Autodesk Inventor part; units mm, degrees
ref_plane "YZ Plane" through (0, 0, 0) normal (1, 0, 0) x (0, 1, 0)
ref_plane "XZ Plane" through (0, 0, 0) normal (0, 1, 0) x (-1, 0, 0)
ref_plane "XY Plane" through (0, 0, 0) normal (0, 0, 1) x (1, 0, 0)
sketch "Szkic1" plane through (0, 0, 0) normal (0, 0, 1) x (1, 0, 0)
  line L0 (-30, -35) -> (30, -35)
  line L1 (30, -35) -> (30, 35)
  line L2 (30, 35) -> (-30, 35)
  line L3 (-30, 35) -> (-30, -35)
  line L4 (-30, -35) -> (30, 35) construction
  line L5 (30, -35) -> (-30, 35) construction
  point P0 (0, 0)
  dimension "d0" = 60
  dimension "d1" = 70
extrude "Wyciągnięcie proste1" add sketch "Szkic1" along normal blind 8
sketch "Szkic2" plane through (0, 0, 0) normal (0, 0, -1) x (-1, 0, 0)
  line L0 (30, -35) -> (-30, -35)
  line L1 (30, 35) -> (30, -35)
  line L2 (-30, 35) -> (30, 35)
  line L3 (-30, -35) -> (-30, 35)
  line L4 (23.57, 5) -> (23.57, 28.57)
  line L5 (23.57, 28.57) -> (-23.57, 28.57)
  line L6 (-23.57, 28.57) -> (-23.57, -18.57)
  line L7 (-23.57, -18.57) -> (23.57, -18.57)
  line L8 (23.57, -18.57) -> (23.57, 5)
  circle A0 centre (23.57, 28.57) radius 2.5
  circle A1 centre (-23.57, 28.57) radius 2.5
  circle A2 centre (-23.57, -18.57) radius 2.5
  circle A3 centre (23.57, -18.57) radius 2.5
  line L9 (0, 0) -> (0, 5)
  dimension "d6" = 47.14
  dimension "d7" = 47.14
  dimension "d8" = 47.14
  dimension "d9" = 5
  dimension "d10" = 5
  dimension "d11" = 5
  dimension "d12" = 5
  dimension "d15" = 5
extrude "Wyciągnięcie proste3" cut sketch "Szkic2" against normal up to next contours A0 L5 L4 | L4 L5 A0 | A3 L7 L8 | L8 L7 A3 | A1 L6 L5 | L5 L6 A1 | A2 L6 L7 | L7 L6 A2
sketch "Szkic4" plane through (0, 0, 8) normal (0, 0, 1) x (1, 0, 0)
  line L0 (-30, -35) -> (30, -35)
  line L1 (30, -35) -> (30, -43)
  line L2 (30, -43) -> (-30, -43)
  line L3 (-30, -43) -> (-30, -35)
  point P0 (0, 0)
  dimension "d18" = 8
extrude "Wyciągnięcie proste4" add sketch "Szkic4" against normal blind 43.4
sketch "Szkic5" plane through (0, 0, 8) normal (0, 0, 1) x (1, 0, 0)
  circle A0 centre (-23.57, -18.57) radius 2.5
  circle A1 centre (23.57, 28.57) radius 2.5
  circle A2 centre (-23.57, 28.57) radius 2.5
  circle A3 centre (23.57, -18.57) radius 2.5
  line L0 (30, 35) -> (30, -43)
  line L1 (30, 35) -> (-30, 35)
  line L2 (-30, 35) -> (-30, -43)
  line L3 (30, -43) -> (-30, -43)
  line L4 (23.57, -18.57) -> (-23.57, 28.57)
  line L5 (-23.57, -18.57) -> (23.57, 28.57)
  circle A4 centre (0, 5) radius 15
  point P0 (0, 0)
  dimension "d21" = 30
extrude "Wyciągnięcie proste5" cut sketch "Szkic5" against normal up to next contours A4 L4 L5 | L5 L4 A4 | L5 A4 L4 | L4 A4 L5
thread "Gwint1"
thread "Gwint2"
thread "Gwint3"
thread "Gwint4"
sketch "Szkic10" plane through (0, 0, 0) normal (0, 0, -1) x (-1, 0, 0)
  circle A0 centre (0, 5) radius 15
  circle A1 centre (0, 5) radius 19.5
  point P0 (0, 0)
  dimension "d59" = 39
extrude "Wyciągnięcie proste10" cut sketch "Szkic10" against normal blind 2
sketch "Szkic12" plane through (0, 0, -35.4) normal (0, 0, -1) x (-1, 0, 0)
  line L0 (30, -35) -> (-30, -35)
  line L1 (-30, -35) -> (-30, -43)
  line L2 (-30, -43) -> (30, -43)
  line L3 (30, -43) -> (30, -35)
  point P0 (0, 0)
extrude "Wyciągnięcie proste12" cut sketch "Szkic12" against normal blind 20
sketch "Szkic13" plane through (-30, -43, 8) normal (0, -1, 0) x (1, 0, 0)
  line L0 (0, -23.4) -> (60, -23.4)
  line L1 (0, 0) -> (0, -23.4)
  line L2 (60, 0) -> (60, -23.4)
  line L3 (60, -23.4) -> (60, -15.4)
  line L4 (60, -8) -> (60, -23.4)
  line L5 (60, -15.4) -> (0, -15.4)
  point P0 (30, -8)
  dimension "d66" = 8
extrude "Wyciągnięcie proste13" add sketch "Szkic13" along normal blind 60
sketch "Szkic16" plane through (-30, -43, -7.4) normal (0, 0, 1) x (1, 0, 0)
  line L0 (60, -60) -> (0, -60)
  line L1 (60, 0) -> (60, -60)
  line L2 (0, 0) -> (60, 0)
  line L3 (0, 0) -> (0, -60)
  circle A0 centre (30, -20) radius 6.5
  line L4 (30, -20) -> (35, -20)
  line L5 (30, -20) -> (25, -20)
  arc A1 (35, -30) -> (35, -10) centre (35, -20) ccw
  arc A2 (25, -10) -> (25, -30) centre (25, -20) ccw
  line L6 (25, -10) -> (35, -10)
  line L7 (35, -30) -> (25, -30)
  point P0 (30, 43)
  dimension "d87" = 5
  dimension "d88" = 5
  dimension "d89" = 10
extrude "Wyciągnięcie proste15" cut sketch "Szkic16" against normal up to next contours A0 | L7 A2 L6 A1
sketch "Szkic17" plane through (-30, -43, -7.4) normal (0, 0, 1) x (1, 0, 0)
  line L0 (25, -10) -> (35, -10)
  arc A0 (35, -30) -> (35, -10) centre (35, -20) ccw
  line L1 (35, -30) -> (25, -30)
  arc A1 (25, -10) -> (25, -30) centre (25, -20) ccw
  line L2 (0, 0) -> (60, 0)
  line L3 (0, 0) -> (0, -60)
  line L4 (60, -60) -> (0, -60)
  line L5 (60, 0) -> (60, -60)
  line L6 (60, 0) -> (60, -5)
  line L7 (60, 8) -> (60, -60)
  line L8 (30, -30) -> (30, -35)
  line L9 (60, -5) -> (57.5, -5)
  arc A2 (55, -7.5) -> (55, -2.5) centre (55, -5) ccw
  arc A3 (45, -2.5) -> (45, -7.5) centre (45, -5) ccw
  line L10 (55, -7.5) -> (45, -7.5)
  line L11 (60, -5) -> (57.5, -5)
  line L12 (55, -2.5) -> (45, -2.5)
  line L13 (60, -35) -> (57.5, -35)
  arc A4 (55, -37.5) -> (55, -32.5) centre (55, -35) ccw
  arc A5 (45, -32.5) -> (45, -37.5) centre (45, -35) ccw
  line L14 (55, -37.5) -> (45, -37.5)
  line L15 (55, -32.5) -> (45, -32.5)
  line L16 (30, -35) -> (42.5, -35)
  line L17 (57.5, -35) -> (60, -35)
  line L18 (0, -5) -> (2.5, -5)
  line L19 (0, -35) -> (2.5, -35)
  arc A6 (15, -7.5) -> (15, -2.5) centre (15, -5) ccw
  line L20 (15, -7.5) -> (5, -7.5)
  line L21 (15, -2.5) -> (5, -2.5)
  arc A7 (5, -2.5) -> (5, -7.5) centre (5, -5) ccw
  arc A8 (15, -37.5) -> (15, -32.5) centre (15, -35) ccw
  line L22 (15, -37.5) -> (5, -37.5)
  line L23 (15, -32.5) -> (5, -32.5)
  arc A9 (5, -32.5) -> (5, -37.5) centre (5, -35) ccw
  line L24 (42.5, -5) -> (17.5, -5)
  line L25 (2.5, -5) -> (0, -5)
  line L26 (30, -35) -> (17.5, -35)
  line L27 (2.5, -35) -> (0, -35)
  point P0 (30, 43)
  dimension "d92" = 5
  dimension "d93" = 5
  dimension "d98" = 2.5
  dimension "d99" = 2.5
  dimension "d100" = 2.5
  dimension "d101" = 2.5
extrude "Wyciągnięcie proste16" cut sketch "Szkic17" against normal up to next contours A5 L15 A4 L14 | A8 L22 A9 L23 | A2 L10 A3 L12 | A7 L21 A6 L20
sketch "Szkic18" plane through (-30, -43, -7.4) normal (0, 0, 1) x (1, 0, 0)
  line L0 (55, -5) -> (50, -5)
  line L1 (55, -35) -> (50, -35)
  line L2 (5, -5) -> (10, -5)
  line L3 (5, -35) -> (10, -35)
  circle A0 centre (10, -5) radius 2
  circle A1 centre (10, -35) radius 2
  circle A2 centre (50, -35) radius 2
  circle A3 centre (50, -5) radius 2
  line L4 (45, -2.5) -> (55, -2.5)
  arc A4 (55, -7.5) -> (55, -2.5) centre (55, -5) ccw
  line L5 (55, -7.5) -> (45, -7.5)
  arc A5 (45, -2.5) -> (45, -7.5) centre (45, -5) ccw
  line L6 (15, -37.5) -> (5, -37.5)
  arc A6 (5, -32.5) -> (5, -37.5) centre (5, -35) ccw
  line L7 (5, -32.5) -> (15, -32.5)
  arc A7 (15, -37.5) -> (15, -32.5) centre (15, -35) ccw
  line L8 (5, -2.5) -> (15, -2.5)
  arc A8 (15, -7.5) -> (15, -2.5) centre (15, -5) ccw
  line L9 (15, -7.5) -> (5, -7.5)
  arc A9 (5, -2.5) -> (5, -7.5) centre (5, -5) ccw
  line L10 (55, -37.5) -> (45, -37.5)
  arc A10 (45, -32.5) -> (45, -37.5) centre (45, -35) ccw
  line L11 (45, -32.5) -> (55, -32.5)
  arc A11 (55, -37.5) -> (55, -32.5) centre (55, -35) ccw
  line L12 (25, -10) -> (35, -10)
  arc A12 (35, -30) -> (35, -10) centre (35, -20) ccw
  line L13 (35, -30) -> (25, -30)
  arc A13 (25, -10) -> (25, -30) centre (25, -20) ccw
  line L14 (0, 0) -> (60, 0)
  line L15 (0, 0) -> (0, -60)
  line L16 (60, -60) -> (0, -60)
  line L17 (60, 0) -> (60, -60)
  line L18 (55, -5) -> (60, -5)
  line L19 (55, -35) -> (60, -35)
  line L20 (5, -5) -> (0, -5)
  line L21 (5, -35) -> (0, -35)
  point P0 (30, 43)
  dimension "d104" = 5
  dimension "d105" = 5
  dimension "d106" = 5
  dimension "d107" = 5
  dimension "d108" = 4
  dimension "d109" = 4
  dimension "d110" = 4
  dimension "d111" = 4
sketch "Szkic19" plane through (-30, -43, -7.4) normal (0, 0, 1) x (1, 0, 0)
  line L0 (45, -2.5) -> (55, -2.5)
  arc A0 (55, -7.5) -> (55, -2.5) centre (55, -5) ccw
  line L1 (55, -7.5) -> (45, -7.5)
  arc A1 (45, -2.5) -> (45, -7.5) centre (45, -5) ccw
  line L2 (15, -37.5) -> (5, -37.5)
  arc A2 (5, -32.5) -> (5, -37.5) centre (5, -35) ccw
  line L3 (5, -32.5) -> (15, -32.5)
  arc A3 (15, -37.5) -> (15, -32.5) centre (15, -35) ccw
  line L4 (5, -2.5) -> (15, -2.5)
  arc A4 (15, -7.5) -> (15, -2.5) centre (15, -5) ccw
  line L5 (15, -7.5) -> (5, -7.5)
  arc A5 (5, -2.5) -> (5, -7.5) centre (5, -5) ccw
  line L6 (55, -37.5) -> (45, -37.5)
  arc A6 (45, -32.5) -> (45, -37.5) centre (45, -35) ccw
  line L7 (45, -32.5) -> (55, -32.5)
  arc A7 (55, -37.5) -> (55, -32.5) centre (55, -35) ccw
  line L8 (25, -10) -> (35, -10)
  arc A8 (35, -30) -> (35, -10) centre (35, -20) ccw
  line L9 (35, -30) -> (25, -30)
  arc A9 (25, -10) -> (25, -30) centre (25, -20) ccw
  line L10 (0, 0) -> (60, 0)
  line L11 (60, -60) -> (0, -60)
  line L12 (60, 0) -> (60, -60)
  line L13 (60, 0) -> (60, -60)
  line L14 (60, -60) -> (0, -60)
  line L15 (0, 0) -> (60, 0)
  circle A10 centre (29.9999, -20) radius 6.5
  circle A11 centre (-10.0001, -20) radius 6.5
  line L16 (-10.0001, -20) -> (-5.0001, -20)
  arc A12 (0, -28.6602) -> (0, -11.3398) centre (-5.0001, -20) ccw
  line L17 (0, 0) -> (0, -2.5)
  line L18 (0, -37.5) -> (0, -60)
  line L19 (0, -11.3398) -> (0, -2.5)
  line L20 (0, 8) -> (0, -60)
  line L21 (0, -28.6602) -> (0, -37.5)
  line L22 (-5.0001, -20) -> (-3.5001, -20)
  line L23 (0, -11.3398) -> (-3.5001, -11.3398)
  line L24 (-3.5001, -11.3398) -> (-3.5001, -28.6602)
  line L25 (-3.5001, -28.6602) -> (0, -28.6602)
  point P0 (30, 43)
  dimension "d112" = 13
  dimension "d113" = 13
  dimension "d114" = 4.9999
  dimension "d115" = 5
extrude "Wyciągnięcie proste17" cut sketch "Szkic19" against normal up to next contours A12 L20 | L20 L25 L24 L23
properties part number "Uchwyt silnika krokowego osi X"
Could you check a few things on this model? Use its own coordinates, in mm. A direction names the side the tool comes from. Coordinates: 2 decimals unless noted, no trailing zeros. Order: outer loops, then holes, each group sorted by start corner. A loop starts at its lowest first (then second) coordinate and runs counter-clockwise, first axis right, second up. Notation, with made-up numbers: M 52,73.5 L 91,73.5 A20 ccw 91,81.5 Z; hole C 69,-35 d9. An arc over 180 degrees is marked long. Use one line per item in the form item = value. Start each with the question number.
1. Suppose I cut it at C-C on y = -78. Write out the boundary of the cut face in (x, z), then the cut area to 3 significant figures.
2. Suppose I cut it at B-B on x = 18. Write out the boundary of the cut face in (y, z), then the cut area to 3 significant figures.
3. We'd pull the mould along Y, two halves only. Please class faces 6 (the cylindrical face through (12.5, -77.9, -11.3)), 7 (the flat face through (-20, -80.5, -11)), 8 (the flat face through (0, -43, 0)), 9 (the flat face through (30, -39, -2)): +Y half, -Y half, draft (parallel to the pull), parting line (faces both ways), or undercut.
4. On a 3-axis mill with a long thin cutter (end or side, diameter ignored), from which of +Z, -Z, +X, -X, +Y, -Y can I reach the whole of each face in a straight line? I mean faces 1 (the cylindrical face through (-27.5, -47.9, -11.3)), 2 (the flat face through (0, -12, 8)), 3 (the flat face through (0, -76, -15.4)), 4 (the flat face through (0, -35, -8)), 5 (the flat face through (-10, -6.5, 2)). Say none if no direction works.
5. Suppose I cut it at A-A on y = 5. Write out the boundary of the cut face in (x, z), then the cut area to 3 significant figures.
6. Suppose I cut it at D-D on x = -23.57. Write out the boundary of the cut face in (y, z).
7. Please list where these lines run through material, in increasing order: line 1 (Y direction, x = -23.57, z = 2.25); line 2 (X direction, y = -18.57, z = 6.25); line 3 (Y direction, x = 3, z = -14.5).
8. For pin 1 (5 mm diameter, centred on y = -60.5, z = -12.5, fed in from -X); pin 2 (3 mm diameter, centred on x = 23.57, y = 28.57, fed in from -Z) (3 decimals); pin 3 (6.5 mm diameter, centred on x = 23.57, y = -18.57, fed in from -Z); pin 4 (12.5 mm diameter, centred on x = 15, z = -4.5, fed in from +Y), each with a flat end and sliding along its axis, tell me the tip position at first contact or that it passes through.
Geometry says:
q1.outline = M -30,-15.4 L -27.5,-15.4 L -27.5,-7.4 L -30,-7.4 Z; M -12.5,-15.4 L 12.5,-15.4 L 12.5,-7.4 L -12.5,-7.4 Z; M 27.5,-15.4 L 30,-15.4 L 30,-7.4 L 27.5,-7.4 Z
q1.area = 240 mm^2
q2.outline = M -103,-15.4 L -80.5,-15.4 L -80.5,-7.4 L -103,-7.4 Z; M -75.5,-15.4 L -50.5,-15.4 L -50.5,-7.4 L -75.5,-7.4 Z; M -45.5,-15.4 L -35,-15.4 L -35,0 L -2.5,0 L -2.5,2 L 12.5,2 L 12.5,0 L 35,0 L 35,8 L -43,8 L -43,-7.4 L -45.5,-7.4 Z
q2.area = 1,120 mm^2
q3.face_6 = undercut
q3.face_7 = undercut
q3.face_8 = -Y half
q3.face_9 = draft
q4.face_1 = +Z, -Z
q4.face_2 = +Z, +X, -X, +Y, -Y
q4.face_3 = -Z, +X, -X, +Y, -Y
q4.face_4 = -Z, +X, -X, +Y
q4.face_5 = -Z
q5.outline = M -30,0 L -19.5,0 L -19.5,2 L -15,2 L -15,8 L -30,8 Z; M 15,2 L 19.5,2 L 19.5,0 L 30,0 L 30,8 L 15,8 Z
q5.area = 222 mm^2
q6.outline = M -103,-15.4 L -80.5,-15.4 L -80.5,-7.4 L -103,-7.4 Z; M -75.5,-15.4 L -50.5,-15.4 L -50.5,-7.4 L -75.5,-7.4 Z; M -45.5,-15.4 L -35,-15.4 L -35,0 L -21.07,0 L -21.07,8 L -43,8 L -43,-7.4 L -45.5,-7.4 Z; M -16.07,0 L 26.07,0 L 26.07,8 L -16.07,8 Z; M 31.07,0 L 35,0 L 35,8 L 31.07,8 Z
q7.line_1 = -43 to -21.07, -16.07 to 26.07, 31.07 to 35
q7.line_2 = -30 to -26.07, -21.07 to 21.07, 26.07 to 30
q7.line_3 = -103 to -73, -53 to -35
q8.pin_1 = -26.34
q8.pin_2 = through
q8.pin_3 = 0
q8.pin_4 = 35
